Geometry: final body of the model. Coordinates: model frame, mm. Round coordinates to 2 decimals unless told otherwise and drop trailing zeros. Write each loop counter-clockwise with the first axis right and the second up, starting at its lowest first coordinate (ties: lowest second). Pieces come first, ordered by that corner, then holes. Notation, with made-up numbers: M 43,-12 L 75,-12 A23 ccw 75,10 Z; hole C 21,46.25 d6. An arc over 180 degrees is marked long. Put each result on its own line as item: value. Start each with the question number.
```python
from build123d import *

# Parameters (mm, degrees)
SKETCH_1_R               = 1.5
SKETCH_1_R_2             = 9
EXTRUDE_1_DEPTH          = 2
CUT_EXTRUDE_1_DEPTH      = 100.85333965
CUT_EXTRUDE_1_DEPTH_BACK = 100.85333965
SKETCH_2_R               = 1.5
CUT_EXTRUDE_2_DEPTH      = 100.85333965
CUT_EXTRUDE_2_DEPTH_BACK = 100.85333965


with BuildPart() as part:
    # 草图1 → 凸台-拉伸1 (new body)
    with BuildSketch(Plane(origin=(0, 0, 0), x_dir=(1, 0, 0), z_dir=(0, 1, 0))):
        with BuildLine():
            Line((0, 47), (75.321800738, 47))
            ThreePointArc((75.321800738, 47), (76.607375957, 46.532088886), (77.291416244, 45.347296355))
            Line((77.291416244, 45.347296355), (88.047362067, -15.652703645))
            ThreePointArc((88.047362067, -15.652703645), (87.609835447, -17.285575219), (86.077746561, -18))
            Line((86.077746561, -18), (64.077746561, -18))
            ThreePointArc((64.077746561, -18), (48.289235397, -21.406433974), (35.309770387, -31.019673035))
            ThreePointArc((35.309770387, -31.019673035), (-42.818948099, -19.378794691), (0, 47))
        make_face()
        with Locations(Location((-16.264045876, 39.264880132, 0), (0, 0, 270))):
            Circle(SKETCH_1_R, mode=Mode.SUBTRACT)
        with Locations(Location((16.264045876, 39.264880132, 0), (0, 0, 270))):
            Circle(SKETCH_1_R, mode=Mode.SUBTRACT)
        with Locations(Location((39.264880132, -16.264045876, 0), (0, 0, 270))):
            Circle(SKETCH_1_R, mode=Mode.SUBTRACT)
        with Locations(Location((16.264045876, -39.264880132, 0), (0, 0, 270))):
            Circle(SKETCH_1_R, mode=Mode.SUBTRACT)
        with Locations(Location((-16.264045876, -39.264880132, 0), (0, 0, 270))):
            Circle(SKETCH_1_R, mode=Mode.SUBTRACT)
        with Locations(Location((-39.264880132, -16.264045876, 0), (0, 0, 270))):
            Circle(SKETCH_1_R, mode=Mode.SUBTRACT)
        with Locations(Location((-39.264880132, 16.264045876, 0), (0, 0, 270))):
            Circle(SKETCH_1_R, mode=Mode.SUBTRACT)
        with Locations(Location((0, 0, 0), (0, 0, 270))):
            Circle(SKETCH_1_R_2, mode=Mode.SUBTRACT)
        with Locations(Location((-6.783865663, 11.75, 0), (0, 0, 270))):
            Circle(SKETCH_1_R, mode=Mode.SUBTRACT)
        with Locations(Location((6.783865663, 11.75, 0), (0, 0, 270))):
            Circle(SKETCH_1_R, mode=Mode.SUBTRACT)
        with Locations(Location((13.567731326, 0, 0), (0, 0, 270))):
            Circle(SKETCH_1_R, mode=Mode.SUBTRACT)
        with Locations(Location((6.783865663, -11.75, 0), (0, 0, 270))):
            Circle(SKETCH_1_R, mode=Mode.SUBTRACT)
        with Locations(Location((-6.783865663, -11.75, 0), (0, 0, 270))):
            Circle(SKETCH_1_R, mode=Mode.SUBTRACT)
        with Locations(Location((-13.567731326, 0, 0), (0, 0, 270))):
            Circle(SKETCH_1_R, mode=Mode.SUBTRACT)
    extrude(amount=EXTRUDE_1_DEPTH)

    # 草图2 → 切除-拉伸1 (cut, two sides: drawn at the far end of the back side and taken through both)
    with BuildSketch(Plane(origin=(0, 2, 0), x_dir=(1, 0, 0), z_dir=(0, 1, 0)).offset(-CUT_EXTRUDE_1_DEPTH_BACK)):
        with Locations(Location((74.70156336, 37, 0), (0, 0, 270))):
            Circle(SKETCH_2_R)
        with Locations(Location((78.668920425, 14.5, 0), (0, 0, 270))):
            Circle(SKETCH_2_R)
        with Locations(Location((82.636277491, -8, 0), (0, 0, 270))):
            Circle(SKETCH_2_R)
        with Locations(Location((38.146205332, 37, 0), (0, 0, 270))):
            Circle(SKETCH_2_R)
        with Locations(Location((46.080919464, -8, 0), (0, 0, 270))):
            Circle(SKETCH_2_R)
        with Locations(Location((42.113562398, 14.5, 0), (0, 0, 270))):
            Circle(SKETCH_2_R)
        with BuildLine():
            Line((64.216309798, 27.359582102), (68.383866062, 3.72419603))
            ThreePointArc((68.383866062, 3.72419603), (63.51690861, -3.226539554), (56.566173025, 1.640417898))
            Line((56.566173025, 1.640417898), (52.398616761, 25.27580397))
            ThreePointArc((52.398616761, 25.27580397), (57.265574214, 32.226539554), (64.216309798, 27.359582102))
        make_face()
    extrude(amount=CUT_EXTRUDE_1_DEPTH + CUT_EXTRUDE_1_DEPTH_BACK, mode=Mode.SUBTRACT)

    # 草图3 → 切除-拉伸2 (cut, two sides: drawn at the far end of the back side and taken through both)
    with BuildSketch(Plane.XZ.offset(-CUT_EXTRUDE_2_DEPTH_BACK)):
        with BuildLine():
            ThreePointArc((13.035455865, -35.694213682), (23.132934302, -30.147426931), (31.104138605, -21.829625778))
            ThreePointArc((31.104138605, -21.829625778), (31.73567133, -18.668128181), (29.830018752, -16.067668818))
            Line((29.830018752, -16.067668818), (21.121590627, -11.039855496))
            ThreePointArc((21.121590627, -11.039855496), (18.33030278, -10.583005244), (15.934658856, -12.086630926))
            ThreePointArc((15.934658856, -12.086630926), (12.17522858, -15.867066806), (7.550595775, -18.519948797))
            ThreePointArc((7.550595775, -18.519948797), (5.478166623, -20.44479617), (5.197011625, -23.259214737))
            Line((5.197011625, -23.259214737), (7.799599311, -32.972204212))
            ThreePointArc((7.799599311, -32.972204212), (9.818230989, -35.485971662), (13.035455865, -35.694213682))
        make_face()
        with BuildLine():
            ThreePointArc((37.429823749, -6.558070912), (37.674904732, 4.959995304), (34.457079782, 16.022161306))
            ThreePointArc((34.457079782, 16.022161306), (32.03490891, 18.149833488), (28.830018752, 17.799719626))
            Line((28.830018752, 17.799719626), (20.121590627, 12.771906304))
            ThreePointArc((20.121590627, 12.771906304), (18.33030278, 10.583005244), (18.434658856, 7.756503907))
            ThreePointArc((18.434658856, 7.756503907), (19.828897227, 2.610523844), (19.814044022, -2.720966644))
            ThreePointArc((19.814044022, -2.720966644), (20.44479617, -5.478166623), (22.741576647, -7.128863277))
            Line((22.741576647, -7.128863277), (32.454566122, -9.731450963))
            ThreePointArc((32.454566122, -9.731450963), (35.640868431, -9.240148374), (37.429823749, -6.558070912))
        make_face()
        with BuildLine():
            ThreePointArc((24.394367884, 29.13614277), (14.54197043, 35.107422235), (3.352941176, 37.851787084))
            ThreePointArc((3.352941176, 37.851787084), (0.29923758, 36.817961668), (-1, 33.867388444))
            Line((-1, 33.867388444), (-1, 23.8117618))
            ThreePointArc((-1, 23.8117618), (0, 21.166010489), (2.5, 19.843134833))
            ThreePointArc((2.5, 19.843134833), (7.653668647, 18.47759065), (12.263448247, 15.798982153))
            ThreePointArc((12.263448247, 15.798982153), (14.966629547, 14.966629547), (17.544565022, 16.130351459))
            Line((17.544565022, 16.130351459), (24.654966811, 23.240753248))
            ThreePointArc((24.654966811, 23.240753248), (25.822637443, 26.245823287), (24.394367884, 29.13614277))
        make_face()
        with BuildLine():
            ThreePointArc((-13.035455865, 35.694213682), (-23.132934302, 30.147426931), (-31.104138605, 21.829625778))
            ThreePointArc((-31.104138605, 21.829625778), (-31.73567133, 18.668128181), (-29.830018752, 16.067668818))
            Line((-29.830018752, 16.067668818), (-21.121590627, 11.039855496))
            ThreePointArc((-21.121590627, 11.039855496), (-18.33030278, 10.583005244), (-15.934658856, 12.086630926))
            ThreePointArc((-15.934658856, 12.086630926), (-12.17522858, 15.867066806), (-7.550595775, 18.519948797))
            ThreePointArc((-7.550595775, 18.519948797), (-5.478166623, 20.44479617), (-5.197011625, 23.259214737))
            Line((-5.197011625, 23.259214737), (-7.799599311, 32.972204212))
            ThreePointArc((-7.799599311, 32.972204212), (-9.818230989, 35.485971662), (-13.035455865, 35.694213682))
        make_face()
        with BuildLine():
            ThreePointArc((-37.429823749, 6.558070912), (-37.674904732, -4.959995304), (-34.457079782, -16.022161306))
            ThreePointArc((-34.457079782, -16.022161306), (-32.03490891, -18.149833488), (-28.830018752, -17.799719626))
            Line((-28.830018752, -17.799719626), (-20.121590627, -12.771906304))
            ThreePointArc((-20.121590627, -12.771906304), (-18.33030278, -10.583005244), (-18.434658856, -7.756503907))
            ThreePointArc((-18.434658856, -7.756503907), (-19.828897227, -2.610523844), (-19.814044022, 2.720966644))
            ThreePointArc((-19.814044022, 2.720966644), (-20.44479617, 5.478166623), (-22.741576647, 7.128863277))
            Line((-22.741576647, 7.128863277), (-32.454566122, 9.731450963))
            ThreePointArc((-32.454566122, 9.731450963), (-35.640868431, 9.240148374), (-37.429823749, 6.558070912))
        make_face()
        with BuildLine():
            ThreePointArc((-24.394367884, -29.13614277), (-14.54197043, -35.107422235), (-3.352941176, -37.851787084))
            ThreePointArc((-3.352941176, -37.851787084), (-0.29923758, -36.817961668), (1, -33.867388444))
            Line((1, -33.867388444), (1, -23.8117618))
            ThreePointArc((1, -23.8117618), (0, -21.166010489), (-2.5, -19.843134833))
            ThreePointArc((-2.5, -19.843134833), (-7.653668647, -18.47759065), (-12.263448247, -15.798982153))
            ThreePointArc((-12.263448247, -15.798982153), (-14.966629547, -14.966629547), (-17.544565022, -16.130351459))
            Line((-17.544565022, -16.130351459), (-24.654966811, -23.240753248))
            ThreePointArc((-24.654966811, -23.240753248), (-25.822637443, -26.245823287), (-24.394367884, -29.13614277))
        make_face()
    extrude(amount=CUT_EXTRUDE_2_DEPTH + CUT_EXTRUDE_2_DEPTH_BACK, mode=Mode.SUBTRACT)


solid = part.part
```
1) Section B-B, the plane y = 1.5. Give the number of separate pieces and of enclosed holes in the cut face, and give its area (3 significant figures).
2) Section A-A, the plane z = 0. Output: boundary loops of the cut face in (x, y), and give its area (3 significant figures).
3) Draft query along Z for faces 1 (the face through (-6.48, 1.01, 28.05)), 2 (the face through (36, 2, -11)), 3 (the face through (-0.334, 1.014, -36.849)). Return one class per face: +Z half, -Z half, draft (parallel to the pull), parting line (faces both ways), or undercut.
4) First-contact query: pin 1 (0.6 mm diameter, centred on y = 1.5, z = -27.5, fed in from -X). Flat tip, straight axial feed; report the tip coordinate or a pass-through.
5) Ray query, probe 1 along X at (y, z) = (1.3, 40); probe 2 along X at (y, z) = (0.25, -28.5); probe 3 along X at (y, z) = (0.5, 11). Return the intervals inside material, ascending.
Solved:
1. separate pieces: 1
1. enclosed holes: 27
1. area: 6,430 mm2
2. outline: M -47,0 L -38,0 L -38,2 L -47,2 Z; M -20,0 L -15.07,0 L -15.07,2 L -20,2 Z; M -12.07,0 L -9,0 L -9,2 L -12.07,2 Z; M 9,0 L 12.07,0 L 12.07,2 L 9,2 Z; M 15.07,0 L 20,0 L 20,2 L 15.07,2 Z; M 38,0 L 57.11,0 L 57.11,2 L 38,2 Z; M 67.84,0 L 85.29,0 L 85.29,2 L 67.84,2 Z
2. area: 123 mm2
3. face 1: undercut
3. face 2: draft
3. face 3: undercut
4. pin 1: stops at x = -38.33
5. probe 1: x = -24.68 to -17.57, -14.96 to 14.96, 17.57 to 24.68
5. probe 2: x = -37.37 to -25, 1 to 6.6, 25.13 to 52.72, 63.9 to 80.26
5. probe 3: x = -45.69 to -21.05, -17.19 to -8.08, -5.48 to 5.48, 8.08 to 18.5, 36.37 to 87.23
